```python
from build123d import *

# Parameters (mm, degrees)
SKETCH1_R           = 7.9375
SKETCH1_R_2         = 3.2639
BOSS_EXTRUDE1_DEPTH = 6.35
SKETCH2_R           = 14.2875
SKETCH2_R_2         = 2
SKETCH2_R_3         = 8.7503
CUT_EXTRUDE1_DEPTH  = 88.034521299


with BuildPart() as part:
    # Sketch1 → Boss-Extrude1 (new body)
    # profile 1 of 7: a face of its own
    with BuildSketch(Plane(origin=(0, 0, 0), x_dir=(0, 0, -1), z_dir=(1, 0, 0))):
        with BuildLine():
            ThreePointArc((-41.555851826, 28.575), (-49.493351826, 20.6375), (-57.430851826, 28.575))
            Line((-57.430851826, 28.575), (-57.430851826, -28.575))
            ThreePointArc((-57.430851826, -28.575), (-49.493351826, -20.6375), (-41.555851826, -28.575))
            ThreePointArc((-41.555851826, -28.575), (-45.524601826, -35.449076643), (-53.462101826, -35.449076643))
            Line((-53.462101826, -35.449076643), (-3.96875, -64.024076643))
            ThreePointArc((-3.96875, -64.024076643), (-3.96875, -50.275923357), (7.9375, -57.15))
            ThreePointArc((7.9375, -57.15), (6.874076643, -61.11875), (3.96875, -64.024076643))
            Line((3.96875, -64.024076643), (53.462101826, -35.449076643))
            ThreePointArc((53.462101826, -35.449076643), (42.619275184, -24.60625), (57.430851826, -28.575))
            Line((57.430851826, -28.575), (57.430851826, 28.575))
            ThreePointArc((57.430851826, 28.575), (42.619275184, 24.60625), (53.462101826, 35.449076643))
            Line((53.462101826, 35.449076643), (3.96875, 64.024076643))
            ThreePointArc((3.96875, 64.024076643), (6.874076643, 61.11875), (7.9375, 57.15))
            ThreePointArc((7.9375, 57.15), (-3.96875, 50.275923357), (-3.96875, 64.024076643))
            Line((-3.96875, 64.024076643), (-53.462101826, 35.449076643))
            ThreePointArc((-53.462101826, 35.449076643), (-45.524601826, 35.449076643), (-41.555851826, 28.575))
        make_face()
    # profile 2 of 7: a face of its own
    with BuildSketch(Plane(origin=(0, 0, 0), x_dir=(0, 0, -1), z_dir=(1, 0, 0))):
        with Locations((-49.493351826, 28.575)):
            Circle(SKETCH1_R)
        with Locations((-49.493351826, 28.575)):
            Circle(SKETCH1_R_2, mode=Mode.SUBTRACT)
    # profile 3 of 7: a face of its own
    with BuildSketch(Plane(origin=(0, 0, 0), x_dir=(0, 0, -1), z_dir=(1, 0, 0))):
        with Locations((-49.493351826, -28.575)):
            Circle(SKETCH1_R)
        with Locations((-49.493351826, -28.575)):
            Circle(SKETCH1_R_2, mode=Mode.SUBTRACT)
    # profile 4 of 7: a face of its own
    with BuildSketch(Plane(origin=(0, 0, 0), x_dir=(0, 0, -1), z_dir=(1, 0, 0))):
        with Locations((0, 57.15)):
            Circle(SKETCH1_R)
        with Locations((0, 57.15)):
            Circle(SKETCH1_R_2, mode=Mode.SUBTRACT)
    # profile 5 of 7: a face of its own
    with BuildSketch(Plane(origin=(0, 0, 0), x_dir=(0, 0, -1), z_dir=(1, 0, 0))):
        with Locations((49.493351826, 28.575)):
            Circle(SKETCH1_R)
        with Locations((49.493351826, 28.575)):
            Circle(SKETCH1_R_2, mode=Mode.SUBTRACT)
    # profile 6 of 7: a face of its own
    with BuildSketch(Plane(origin=(0, 0, 0), x_dir=(0, 0, -1), z_dir=(1, 0, 0))):
        with Locations((49.493351826, -28.575)):
            Circle(SKETCH1_R)
        with Locations((49.493351826, -28.575)):
            Circle(SKETCH1_R_2, mode=Mode.SUBTRACT)
    # profile 7 of 7: a face of its own
    with BuildSketch(Plane(origin=(0, 0, 0), x_dir=(0, 0, -1), z_dir=(1, 0, 0))):
        with Locations((0, -57.15)):
            Circle(SKETCH1_R)
        with Locations((0, -57.15)):
            Circle(SKETCH1_R_2, mode=Mode.SUBTRACT)
    extrude(amount=BOSS_EXTRUDE1_DEPTH)

    # Sketch2 → Cut-Extrude1 (cut, through all)
    with BuildSketch(Plane(origin=(0, 0, 0), x_dir=(0, 0, -1), z_dir=(1, 0, 0))):
        Circle(SKETCH2_R)
        with Locations((-34.785312841, -31.243129198)):
            Circle(SKETCH2_R_2)
        with Locations((-22.225, -38.494829198)):
            Circle(SKETCH2_R_3)
        with Locations((-9.664687159, -45.746529198)):
            Circle(SKETCH2_R_2)
        with Locations((9.664687159, -45.746529198)):
            Circle(SKETCH2_R_2)
        with Locations((34.785312841, -31.243129198)):
            Circle(SKETCH2_R_2)
        with Locations((22.225, -38.494829198)):
            Circle(SKETCH2_R_3)
        with Locations((44.45, -14.5034)):
            Circle(SKETCH2_R_2)
        with Locations((44.45, 0)):
            Circle(SKETCH2_R_3)
        with Locations((44.45, 14.5034)):
            Circle(SKETCH2_R_2)
        with Locations((34.785312841, 31.243129198)):
            Circle(SKETCH2_R_2)
        with Locations((9.664687159, 45.746529198)):
            Circle(SKETCH2_R_2)
        with Locations((-9.664687159, 45.746529198)):
            Circle(SKETCH2_R_2)
        with Locations((22.225, 38.494829198)):
            Circle(SKETCH2_R_3)
        with Locations((-34.785312841, 31.243129198)):
            Circle(SKETCH2_R_2)
        with Locations((-22.225, 38.494829198)):
            Circle(SKETCH2_R_3)
        with Locations((-44.45, -14.5034)):
            Circle(SKETCH2_R_2)
        with Locations((-44.45, 14.5034)):
            Circle(SKETCH2_R_2)
        with Locations((-44.45, 0)):
            Circle(SKETCH2_R_3)
    extrude(amount=CUT_EXTRUDE1_DEPTH, mode=Mode.SUBTRACT)


solid = part.part
```
Can you work these out from the model? Positions are in its coordinate system, mm. Give positions to 0.01 mm unless a question says otherwise; leave off trailing zeros. Loops run counter-clockwise (first coordinate to the right, second up) from the corner with the lowest first, then second, coordinate; pieces in that order, holes last. Notation, with made-up numbers: M -33.5,22 L -3.5,22 A22 ccw -3.5,54 Z; hole C -8,52 d3. An arc over 180 degrees is marked long. Use one line per item in the form item = value. Start each with the question number.
(1) I want a section at B-B, the plane y = 0. Write out the boundary of the cut face in (x, z).
(2) Thinking about a two-plate mould opening in Y: for faces 1 (the cylindrical face through (3.131, 2.628, -52.796)), 2 (the cylindrical face through (3.13, 32.49, -56.4)), 3 (the flat face through (6.35, 15, 1)), 4 (the cylindrical face through (3.131, -53.914, 0.425)), which applies, released by +Y, released by -Y, zero draft, split by the parting line, or undercut?
(3) I want a section at C-C, the plane y = -57.15. Write out the boundary of the cut face in (x, z) (3 decimals).
(4) I want a section at D-D, the plane x = 1.25. State how many separate pieces and enclosed holes the cut face has, and give its area (3 significant figures).
(5) I want a section at A-A, the plane z = 0. Write out the boundary of the cut face in (x, y).
(6) I'm going to push flat-ended pins straight in: P1, Ø2, axis at x = 4.5, z = 15.5, coming from the +Y side; P2, Ø3.5, axis at y = 14.5, z = 44.45, coming from the -X side; P3, Ø3, axis at x = 4, z = 27.5, coming from the -Y side; P4, Ø2, axis at x = 1.5, z = 9.5, coming from the -Y side. Where does each tip first touch, or does it pass through?
(7) Please list where these lines run through material, in increasing order: line 1 (Y direction, x = 4.5, z = -51); line 2 (Y direction, x = 3.25, z = -24.5); line 3 (Y direction, x = 1, z = 48).
Worked out:
q1.outline = M 0,-57.43 L 6.35,-57.43 L 6.35,-53.2 L 0,-53.2 Z; M 0,-35.7 L 6.35,-35.7 L 6.35,-14.29 L 0,-14.29 Z; M 0,14.29 L 6.35,14.29 L 6.35,35.7 L 0,35.7 Z; M 0,53.2 L 6.35,53.2 L 6.35,57.43 L 0,57.43 Z
q2.face_1 = undercut
q2.face_2 = released by +Y
q2.face_3 = zero draft
q2.face_4 = undercut
q3.outline = M 0,-15.875 L 6.35,-15.875 L 6.35,-3.264 L 0,-3.264 Z; M 0,3.264 L 6.35,3.264 L 6.35,15.875 L 0,15.875 Z
q4.separate_pieces = 1
q4.enclosed_holes = 25
q4.area = 8,970 mm²
q5.outline = M 0,-65.09 L 6.35,-65.09 L 6.35,-60.41 L 0,-60.41 Z; M 0,-53.89 L 6.35,-53.89 L 6.35,-14.29 L 0,-14.29 Z; M 0,14.29 L 6.35,14.29 L 6.35,53.89 L 0,53.89 Z; M 0,60.41 L 6.35,60.41 L 6.35,65.09 L 0,65.09 Z
q6.P1 = 57.94
q6.P2 = through
q6.P3 = -51.3
q6.P4 = -61.41
q7.line_1 = -36.87 to -31.47, -25.68 to -5.8, 5.8 to 25.68, 31.47 to 36.87
q7.line_2 = -52.17 to -46.94, -30.05 to 30.05, 46.94 to 52.17
q7.line_3 = -38.6 to -31.48, -25.67 to -8, 8 to 25.67, 31.48 to 38.6
